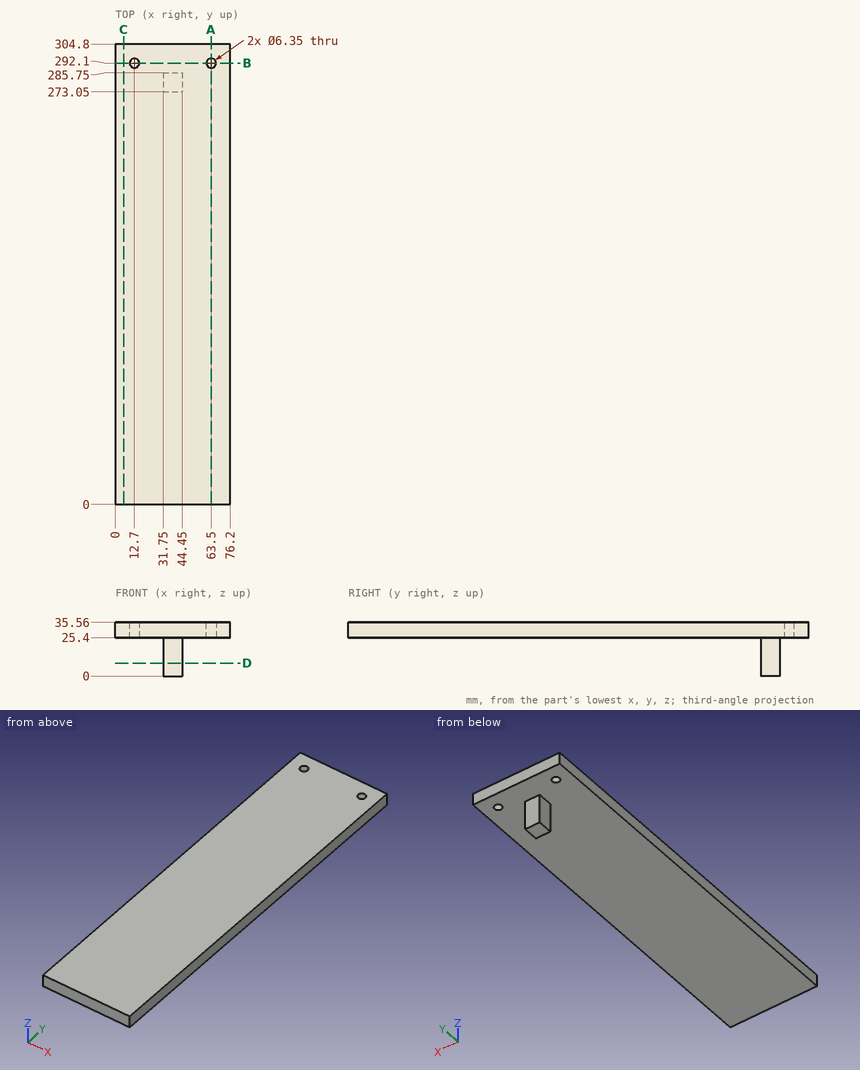
The drawing under review shows one solid part. Ordinate dimensions are in mm from its lowest x, y, z. Give positions to 0.01 mm unless a question says otherwise; leave off trailing zeros. Write each loop counter-clockwise with the first axis right and the second up, starting at its lowest first coordinate (ties: lowest second). Pieces come first, ordered by that corner, then holes. Notation, with made-up numbers: (4.25, 38.25) -> (56.25, 38.25) arc R30 ccw to (56.25, 72.25) -> close; hole circle Ø8 at (0.5, 32.25). An arc over 180 degrees is marked (long way). Put each result on its own line as item: value.
(1) We need section C-C, the plane x = 5.5. Give the boundary of the cut face in (y, z), and give its area (3 significant figures).
Results are:
outline: (0, 25.4) -> (304.8, 25.4) -> (304.8, 35.56) -> (0, 35.56) -> close
area: 3,100 mm²
(2) We need section B-B, the plane y = 292.1. Give the boundary of the cut face in (x, z) (3 decimals).
Results are:
outline: (0, 25.4) -> (9.525, 25.4) -> (9.525, 35.56) -> (0, 35.56) -> close; (15.875, 25.4) -> (60.325, 25.4) -> (60.325, 35.56) -> (15.875, 35.56) -> close; (66.675, 25.4) -> (76.2, 25.4) -> (76.2, 35.56) -> (66.675, 35.56) -> close
(3) We need section D-D, the plane z = 8.5. Give the boundary of the cut face in (x, y), and give its area (3 significant figures).
Results are:
outline: (31.75, 273.05) -> (44.45, 273.05) -> (44.45, 285.75) -> (31.75, 285.75) -> close
area: 161 mm²
(4) To check wall thickness, follow probe 1 along X at (y, z) = (292, 29); probe 2 along Y at (x, z) = (63, 28); probe 3 along Z at (x, y) = (55.5, 58.5). State the ranges of each line that lie inside material, in increasing order. Write a range as from..to.
Results are:
probe 1: 0..9.53, 15.87..60.33, 66.67..76.2
probe 2: 0..288.96, 295.24..304.8
probe 3: 25.4..35.56
(5) For pin 1 Ø3 at (x, z) = (37.5, 17) entering from -Y; pin 2 Ø12 at (x, z) = (59, 20.5) entering from +Y; pin 3 Ø1.5 at (x, y) = (57, 200) entering from -Z; pin 4 Ø4 at (x, z) = (40.5, 9) entering from +Y, all flat-tipped, find the tip position at first contact; note any pin that passes through.
Results are:
pin 1: y = 273.05
pin 2: y = 304.8
pin 3: z = 25.4
pin 4: y = 285.75
(6) We need section A-A, the plane x = 63.5. Give the boundary of the cut face in (y, z) (3 decimals), and give its area (3 significant figures).
Results are:
outline: (0, 25.4) -> (288.925, 25.4) -> (288.925, 35.56) -> (0, 35.56) -> close; (295.275, 25.4) -> (304.8, 25.4) -> (304.8, 35.56) -> (295.275, 35.56) -> close
area: 3,030 mm²
